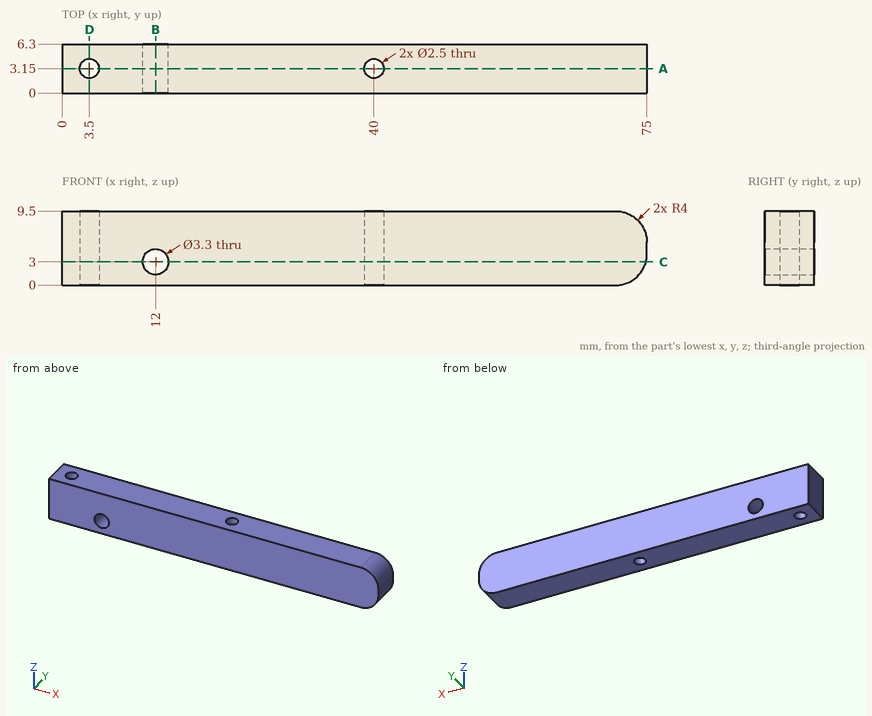
Study the drawing (mm; zero at the part's minimum x, y, z) and answer. Give positions to 0.01 mm unless a question says otherwise; leave off trailing zeros. Order: outer loops, then holes, each group sorted by start corner. A loop starts at its lowest first (then second) coordinate and runs counter-clockwise, first axis right, second up. Notation, with made-up numbers: M -19.5,13 L 20.5,13 A16 cw 20.5,43 Z; hole C 75.5,32.5 d5. An arc over 180 degrees is marked long. Put each result on its own line as item: value. Start each with the question number.
Item 1: The part is cut by section B-B, the plane x = 12. Determine the outline of the cut face in (y, z), and give its area (3 significant figures).
Item 2: Find the intervals of material crossed by line 1 along Y through (x, z) = (40, 8); line 2 along X through (y, z) = (2.5, 2.5); line 3 along X through (y, z) = (3, 6.25), in increasing order.
Item 3: The part is cut by section A-A, the plane y = 3.15. Determine the outline of the cut face in (x, z), and give its area (3 significant figures).
Item 4: The part is cut by section D-D, the plane x = 3.5. Determine the outline of the cut face in (y, z), and give its area (3 significant figures).
Item 5: The part is cut by section C-C, the plane z = 3. Determine the outline of the cut face in (x, y), and give its area (3 significant figures).
Item 6: Flat-ended cylindrical pins translate along their axes: P1, Ø1.5, axis at y = 3, z = 3, coming from the +X side; P2, Ø4.5, axis at x = 12, z = 3, coming from the -Y side. Find the tip coordinate at first contact, or state that the pin passes through.
Answer key:
1. outline: M 0,0 L 6.3,0 L 6.3,1.35 L 0,1.35 Z; M 0,4.65 L 6.3,4.65 L 6.3,9.5 L 0,9.5 Z
1. area: 39.1 mm²
2. line 1: y = 0 to 1.9, 4.4 to 6.3
2. line 2: x = 0 to 2.43, 4.57 to 10.43, 13.57 to 38.93, 41.07 to 74.71
2. line 3: x = 0 to 2.26, 4.74 to 38.76, 41.24 to 74.93
3. outline: M 0,0 L 2.25,0 L 2.25,9.5 L 0,9.5 Z; M 4.75,0 L 38.75,0 L 38.75,9.5 L 4.75,9.5 Z; M 41.25,0 L 71,0 A4 ccw 75,4 L 75,5.5 A4 ccw 71,9.5 L 41.25,9.5 Z; hole C 12,3 d3.3
3. area: 650 mm²
4. outline: M 0,0 L 1.9,0 L 1.9,9.5 L 0,9.5 Z; M 4.4,0 L 6.3,0 L 6.3,9.5 L 4.4,9.5 Z
4. area: 36.1 mm²
5. outline: M 0,0 L 10.35,0 L 10.35,6.3 L 0,6.3 Z; M 13.65,0 L 74.87,0 L 74.87,6.3 L 13.65,6.3 Z; hole C 3.5,3.15 d2.5; hole C 40,3.15 d2.5
5. area: 441 mm²
6. P1: stops at x = 74.99
6. P2: stops at y = 0
